Work out the finished part from the listing and answer in its coordinate system (mm). Give positions to 0.01 mm unless a question says otherwise; leave off trailing zeros. Write each loop counter-clockwise with the first axis right and the second up, starting at its lowest first coordinate (ties: lowest second). Pieces come first, ordered by that corner, then holes.
1) Find section D-D (x = -12.5). Determine the outline of the cut face in (y, z), plus the area to 3 significant figures.
2) Find section B-B (y = -12.7). Determine the outline of the cut face in (x, z), plus the area to 3 significant figures.
3) Straight lines are drawn through the part: probe 1 along X at (y, z) = (-14.5, 22.5); probe 2 along X at (y, z) = (-15.25, -23); probe 3 along Z at (x, y) = (9, -12). For each, find the intervals that lie inside material, in ascending order.
4) Find section A-A (z = 15.5). Determine the outline of the cut face in (x, y).
5) Determine the mould class of faces 1 (the face through (-12.3, 0, -8)), 2 (the face through (-12.3, -25.4, -8)), 3 (the face through (10, -13, 37.989)), 4 (the face through (51.084, -11.628, 0.423)) for opening direction Y: pulls with the +Y half, pulls with the -Y half, needs draft (parallel to the pull), parting line crosses it, or undercut.
6) Given pin 1 Ø1 at (x, z) = (-26, 23) entering from +Y; pin 2 Ø2 at (y, z) = (-18.5, -16) entering from -X, each flat-ended and moving along its own axis, determine where each tip first touches the part or whether it passes through.
7) Find section C-C (x = 26). Determine the outline of the cut face in (y, z).
```python
from build123d import *

# Parameters (mm, degrees)
F1_DEPTH = 25.4
F2_R     = 23.749
F3_DEPTH = 25.401
F4_R     = 3.5687
F5_DEPTH = 76.201


with BuildPart() as f1:
    # F0 (on Front) → F1 (new body)
    with BuildSketch(Plane.XZ):
        Polygon((57.205297, 37.989184), (-38.044703, 37.989184), (-37.823511, -38.210816), (57.205297, -38.210816), align=None)
    extrude(amount=F1_DEPTH)

    # F2 (on face) → F3 (cut, through all)
    with BuildSketch(Plane.XZ.offset(25.4)):
        with Locations((9.453297, 2.302564)):
            Circle(F2_R)
    extrude(amount=-F3_DEPTH, mode=Mode.SUBTRACT)

    # F4 (on face) → F5 (cut, through all)
    with BuildSketch(Plane.XY.offset(37.989184)):
        with Locations((-28.519703, -12.7)):
            Circle(F4_R)
        with Locations((47.680297, -12.7)):
            Circle(F4_R)
    extrude(amount=-F5_DEPTH, mode=Mode.SUBTRACT)


solid = f1.part
```
Results:
1. outline: (-25.4, -38.21) - (0, -38.21) - (0, -6.76) - (-25.4, -6.76) - close; (-25.4, 11.36) - (0, 11.36) - (0, 37.99) - (-25.4, 37.99) - close
1. area: 1,480 mm2
2. outline: (-38.04, 37.99) - (-37.82, -38.21) - (-32.09, -38.21) - (-32.09, 37.99) - close; (-24.95, -38.21) - (44.11, -38.21) - (44.11, 37.99) - (-24.95, 37.99) - close; (51.25, -38.21) - (57.21, -38.21) - (57.21, 37.99) - (51.25, 37.99) - close; hole circle Ø47.5 at (9.45, 2.3)
2. area: 4,390 mm2
3. probe 1: x = -38 to -31.6, -25.44 to -3.04, 21.95 to 44.6, 50.76 to 57.21
3. probe 2: x = -37.87 to -31.02, -26.02 to 45.18, 50.18 to 57.21
3. probe 3: z = -38.21 to -21.44, 26.05 to 37.99
4. outline: (-37.98, -25.4) - (-10.29, -25.4) - (-10.29, 0) - (-37.98, 0) - close; (29.2, -25.4) - (57.21, -25.4) - (57.21, 0) - (29.2, 0) - close; hole circle Ø7.14 at (-28.52, -12.7); hole circle Ø7.14 at (47.68, -12.7)
5. face 1: pulls with the +Y half
5. face 2: pulls with the -Y half
5. face 3: needs draft
5. face 4: undercut
6. pin 1: stops at y = 0
6. pin 2: stops at x = -37.89
7. outline: (-25.4, -38.21) - (0, -38.21) - (0, -14.73) - (-25.4, -14.73) - close; (-25.4, 19.34) - (0, 19.34) - (0, 37.99) - (-25.4, 37.99) - close
